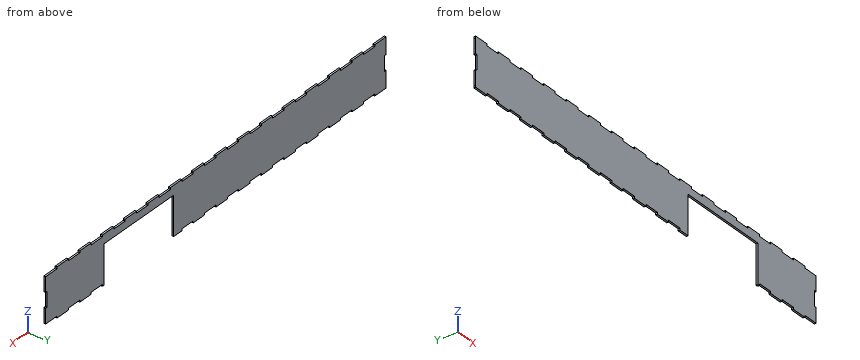
from build123d import *

# Parameters (mm, degrees)
F1_DEPTH = 3.175


# Not quite as in the source:
# - ends of sketch curves that miss each other by under 0.0002 mm in the source are joined


with BuildPart() as f1:
    # F0 (on Front) → F1 (new body)
    with BuildSketch(Plane.XZ):
        Polygon((92.075, 25.4), (244.475, 25.4), (244.475, -38.1), (244.475, -41.2750032454), (247.649968335, -41.2750032454), (247.649968335, -38.1000032454), (272.414968335, -38.1000032454), (272.414968335, -41.2750032454), (297.179968335, -41.2750032454), (297.179968335, -38.1000032454), (321.944968335, -38.1000032454), (321.944968335, -41.2750032454), (346.709968335, -41.2750032453), (346.709968335, -38.1000032454), (371.474968335, -38.0999963909), (371.475, -12.7), (368.3, -12.7), (368.3, 12.7), (371.475, 12.7), (371.475, 38.1), (368.3, 38.1), (346.7100335276, 38.1), (346.7100335276, 41.2750068545), (321.9450335276, 41.2750068544), (321.9450335276, 38.1000068545), (297.1800335276, 38.1000068545), (297.1800335276, 41.2750068545), (272.4150335276, 41.2750068545), (272.4150335276, 38.1000068545), (247.6500335276, 38.1000068545), (247.6500335276, 41.2750068545), (222.8850335276, 41.2750068545), (222.8850335276, 38.1000068545), (198.1200335276, 38.1000068545), (198.1200335276, 41.2750068545), (173.3550335276, 41.2750068545), (173.3550335276, 38.1000068545), (148.5900335276, 38.1000068545), (148.5900335276, 41.2750068545), (123.8250335276, 41.2750068545), (123.8250335276, 38.1000068545), (99.0600335276, 38.1000068545), (99.0600335276, 41.2750068545), (74.2950335276, 41.2750068545), (74.2950335276, 38.1000068545), (49.5300335276, 38.1000068545), (49.5300335276, 41.2750068545), (24.7650335276, 41.2750068545), (24.7650335276, 38.1000068545), (3.35276e-05, 38.1000068545), (3.35276e-05, 41.2750068545), (-24.7649664724, 41.2750068545), (-24.7649664724, 38.1000068545), (-49.5299664724, 38.1000068545), (-49.5299664724, 41.2750068545), (-74.2949664724, 41.2750068545), (-74.2949664724, 38.1000068545), (-99.0599664724, 38.1000068545), (-99.0599664724, 41.2750068545), (-123.8249664724, 41.2750068545), (-123.8249664724, 38.1000068545), (-148.5899664724, 38.1000068545), (-148.5899664724, 41.2750068545), (-173.3549664724, 41.2750068545), (-173.3549664724, 38.1000068545), (-198.1199664724, 38.1000068545), (-198.1199664724, 41.2750068545), (-222.8849664724, 41.2750068545), (-222.8849664724, 38.1000068545), (-247.6499664724, 38.1000068545), (-247.6499664724, 41.2750068545), (-272.4149664724, 41.2750068545), (-272.4149664724, 38.1000068545), (-297.1799664724, 38.1000068545), (-297.1799664724, 41.2750068545), (-321.9449664724, 41.2750068545), (-321.9449664724, 38.1000068545), (-346.7099664724, 38.1000068545), (-346.7099664724, 41.2750068545), (-371.4749664724, 41.2750068545), (-371.475, 38.1), (-371.475, 12.7), (-368.3, 12.7), (-368.3, -12.7), (-371.475, -12.7), (-371.475, -38.1), (-371.475031665, -41.2750032454), (-346.710031665, -41.2750032454), (-346.710031665, -38.1000032454), (-321.945031665, -38.1000032454), (-321.945031665, -41.2750032454), (-297.180031665, -41.2750032454), (-297.180031665, -38.1000032454), (-272.415031665, -38.1000032454), (-272.415031665, -41.2750032454), (-247.650031665, -41.2750032454), (-247.650031665, -38.1000032454), (-222.885031665, -38.1000032454), (-222.885031665, -41.2750032454), (-198.120031665, -41.2750032454), (-198.120031665, -38.1000032454), (-173.355031665, -38.1000032454), (-173.355031665, -41.2750032454), (-148.590031665, -41.2750032454), (-148.590031665, -38.1000032454), (-123.825031665, -38.1000032454), (-123.825031665, -41.2750032454), (-99.060031665, -41.2750032454), (-99.060031665, -38.1000032454), (-74.295031665, -38.1000032454), (-74.295031665, -41.2750032454), (-49.530031665, -41.2750032454), (-49.530031665, -38.1000032454), (-24.765031665, -38.1000032454), (-24.765031665, -41.2750032454), (-3.1665e-05, -41.2750032454), (-3.1665e-05, -38.1000032454), (24.764968335, -38.1000032454), (24.764968335, -41.2750032454), (49.529968335, -41.2750032454), (49.529968335, -38.1000032454), (74.294968335, -38.1000032454), (74.294968335, -41.2750032454), (92.075, -41.2750032454), (92.075, -38.1), align=None)
    extrude(amount=F1_DEPTH)


solid = f1.part
Build history of the part. All positions in model axes, mm. Give positions to 0.01 mm unless a question says otherwise; leave off trailing zeros. Order: outer loops, then holes, each group sorted by start corner. A loop starts at its lowest first (then second) coordinate and runs counter-clockwise, first axis right, second up. Notation, with made-up numbers: M 11.5,-2.75 L 64.5,-2.75 A22 cw 64.5,22.25 Z; hole C 58.25,81 d4. An arc over 180 degrees is marked long. Put each result on its own line as item: value.
Item 1: Drop flat-ended pins along their axis: pin 1 Ø1 at (x, y) = (-89, -1) entering from -Z; pin 2 Ø1 at (y, z) = (-1.5, 40) entering from +X. Give the stop position or say it passes through.
Results are:
pin 1: z = -38.1
pin 2: x = 346.71
Item 2: Cut at B-B on x = 235.5. Write the cut outline in (y, z) (3 decimals).
Results are:
outline: M -3.175,25.4 L 0,25.4 L 0,41.275 L -3.175,41.275 Z
Item 3: Wall check: probe 1 along X at (y, z) = (-2.2, -32) (3 decimals); probe 2 along X at (y, z) = (-1.55, -10.5) (3 decimals); probe 3 along Z at (x, y) = (117.5, -0.7). Give the ranges that are in metal, low to high.
Results are:
probe 1: -371.475 to 92.075, 244.475 to 371.475
probe 2: -368.3 to 92.075, 244.475 to 368.3
probe 3: 25.4 to 38.1
Item 4: Cut at A-A on z = -6.5. Write the cut outline in (x, y) (3 decimals).
Results are:
outline: M -368.3,-3.175 L 92.075,-3.175 L 92.075,0 L -368.3,0 Z; M 244.475,-3.175 L 368.3,-3.175 L 368.3,0 L 244.475,0 Z
